Part model, mm, in its own coordinate system. A direction names the side the tool comes from. Round coordinates to 2 decimals unless told otherwise and drop trailing zeros. Order: outer loops, then holes, each group sorted by start corner. A loop starts at its lowest first (then second) coordinate and runs counter-clockwise, first axis right, second up. Notation, with made-up numbers: M 62.25,-25.75 L 119.25,-25.75 A16 cw 119.25,-7.75 Z; hole C 38.5,35 d4. An arc over 180 degrees is marked long. One line per question, with ' | ' between items.
from build123d import *

# Parameters (mm, degrees)
F0_R     = 19.05
F1_DEPTH = 6.35
F1_TAPER = -30
F2_R     = 1.651
F3_DEPTH = 25.4
F5_DEPTH = 3.175


with BuildPart() as f1:
    # F0 (on Top) → F1 (new body)
    with BuildSketch(Plane.XY):
        Circle(F0_R)
    extrude(amount=-F1_DEPTH, taper=F1_TAPER)

    # F2 (on face) → F3 (cut)
    with BuildSketch(Plane.XY):
        with Locations((0, 12.7)):
            Circle(F2_R)
        with Locations((-10.9985226281, -6.35)):
            Circle(F2_R)
        with Locations((10.9985226281, -6.35)):
            Circle(F2_R)
    extrude(amount=-F3_DEPTH, mode=Mode.SUBTRACT)

    # F4 (on face) → F5 (cut)
    with BuildSketch(Plane(origin=(0, 0, -6.35), x_dir=(1, 0, 0), z_dir=(0, 0, -1))):
        Polygon((4.4170216301, -11.6245720608), (1.2771628997, -8.3370330896), (-3.1398587304, -9.4124610289), (-4.4170216301, -13.7754279392), (-1.2771628997, -17.0629669104), (3.1398587304, -15.9875389711), align=None)
        Polygon((9.7213597283, 1.9870330896), (14.1383813584, 3.0624610289), (15.4155442582, 7.4254279392), (12.2756855278, 10.7129669104), (7.8586638977, 9.6375389711), (6.581500998, 5.2745720608), align=None)
        Polygon((-6.581500998, 7.4254279392), (-9.7213597283, 10.7129669104), (-14.1383813584, 9.6375389711), (-15.4155442582, 5.2745720608), (-12.2756855278, 1.9870330896), (-7.8586638977, 3.0624610289), align=None)
    extrude(amount=-F5_DEPTH, mode=Mode.SUBTRACT)


solid = f1.part
1) Saw through at A-A (x = 0). List the corners of the cut face in (y, z) (3 decimals).
The answers:
outline: M -22.716,-6.35 L 8.648,-6.35 L 8.648,-3.175 L 11.049,-3.175 L 11.049,0 L -19.05,0 Z; M 14.351,-3.175 L 16.752,-3.175 L 16.752,-6.35 L 22.716,-6.35 L 19.05,0 L 14.351,0 Z
2) Drop flat-ended pins along their axis: pin 1 (9.5 mm diameter, centred on x = -13, y = -7.5, fed in from -Z); pin 2 (2.5 mm diameter, centred on x = 10.5, y = -6, fed in from -Z) (3 decimals); pin 3 (1 mm diameter, centred on y = 16.5, z = -4, fed in from -X); pin 4 (1.5 mm diameter, centred on y = 0, z = -4.5, fed in from +X). Give the stop position or say it passes through.
The answers:
pin 1: stops at z = -6.35 | pin 2: stops at z = -3.175 | pin 3: stops at x = -14.3 | pin 4: stops at x = 22.08
3) Two-plate mould, pull along Y, no slides. Class faces 3 (the face through (-11, -8, -2)), 4 (the face through (-4.179, -18.821, -0.397)), 5 (the face through (0, 0, 0)): released by +Y, released by -Y, zero draft, split by the parting line, or undercut.
The answers:
face 3: undercut | face 4: split by the parting line | face 5: zero draft
4) Which spindle directions (+Z, -Z, +X, -X, +Y, -Y) get a long thin tool onto all of the face, cutting with end or side? Do faces 1 (the face through (13.868, -9.046, -4.785)), 2 (the face through (0, 0, -6.35)). Say none if no direction does.
The answers:
face 1: -Z | face 2: -Z, +X, -X, +Y, -Y
5) Probe line 1 (Z direction, x = -12, y = -3) (3 decimals); line 2 (Y direction, x = 11.5, z = -3.25); line 3 (Y direction, x = 0, z = -0.5). List the from-to ranges inside material, lowest first. Write a range as [from, to].
The answers:
line 1: z = [-3.175, 0] | line 2: y = [-17.48, -10.52], [-2.42, 17.48] | line 3: y = [-19.34, 11.05], [14.35, 19.34]
6) Saw through at C-C (y = -6.35). Give the number of separate pieces and of enclosed holes in the cut face, plus the area to 3 significant figures.
The answers:
separate pieces: 3 | enclosed holes: 0 | area: 180 mm²
7) Saw through at B-B (z = -5.5). List the corners of the cut face in (x, y).
The answers:
outline: C 0,0 d44.45; hole M -15.42,-5.27 L -14.14,-9.64 L -9.72,-10.71 L -6.58,-7.43 L -7.86,-3.06 L -12.28,-1.99 Z; hole M -4.42,13.78 L -3.14,9.41 L 1.28,8.34 L 4.42,11.62 L 3.14,15.99 L -1.28,17.06 Z; hole M 6.58,-5.27 L 7.86,-9.64 L 12.28,-10.71 L 15.42,-7.43 L 14.14,-3.06 L 9.72,-1.99 Z
